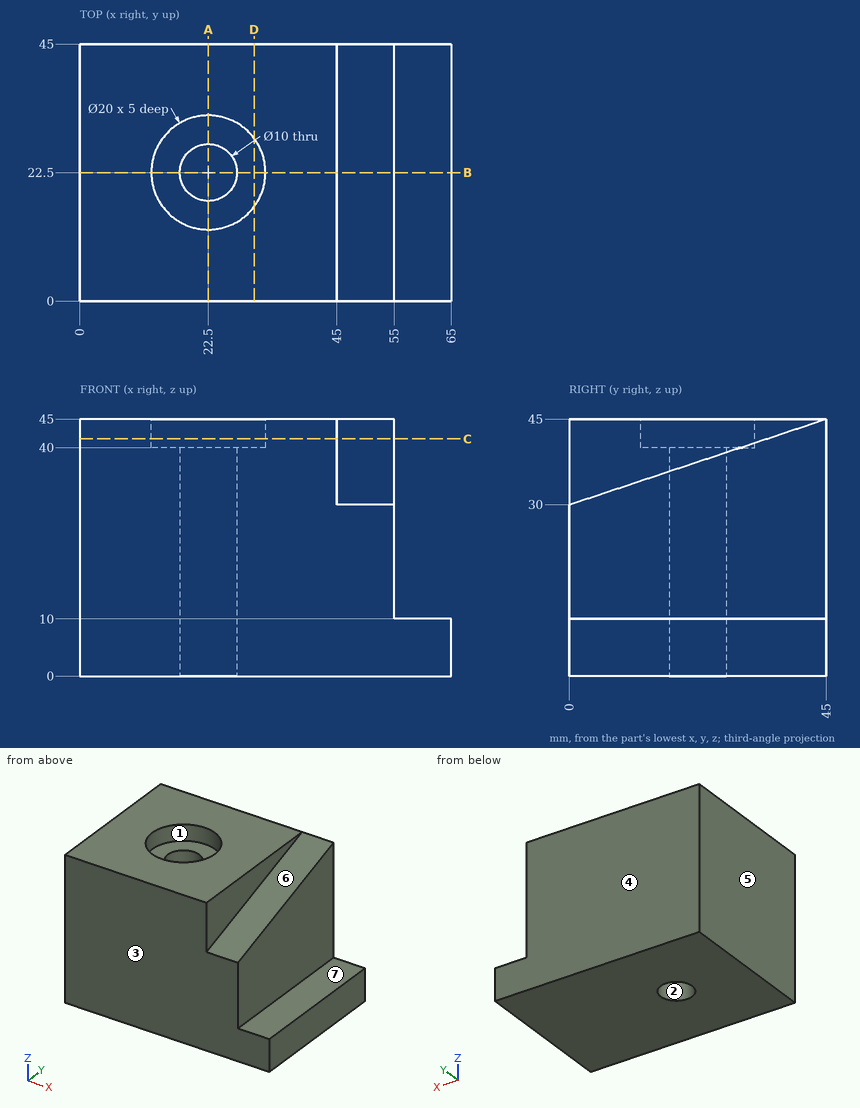
Could you check a few things on this drawing? It's one solid part, dimensions in mm from its lowest x, y, z. A direction names the side the tool comes from. Round coordinates to 2 decimals unless told otherwise and drop trailing zeros. Order: outer loops, then holes, each group sorted by start corner. A loop starts at its lowest first (then second) coordinate and runs counter-clockwise, first axis right, second up. Notation, with made-up numbers: M 87,-37 L 144,-37 A13 ccw 144,-19 Z; hole C -14.75,-33.5 d4. An arc over 180 degrees is marked long. Use a Markdown table: item, result.
1) Imagine slicing it at D-D (x = 30.5). List the corners of the cut face in (y, z) for me, then the cut area to 4 significant figures.
Geometry says:
| item | result |
|---|---|
| outline | M 0,0 L 45,0 L 45,45 L 28.5,45 L 28.5,40 L 16.5,40 L 16.5,45 L 0,45 Z |
| area | 1,965 mm² |
2) Imagine slicing it at A-A (x = 22.5). List the corners of the cut face in (y, z) for me.
Geometry says:
| item | result |
|---|---|
| outline | M 0,0 L 17.5,0 L 17.5,40 L 12.5,40 L 12.5,45 L 0,45 Z; M 27.5,0 L 45,0 L 45,45 L 32.5,45 L 32.5,40 L 27.5,40 Z |
3) On a 3-axis mill with a long thin cutter (end or side, diameter ignored), from which of +Z, -Z, +X, -X, +Y, -Y can I reach the whole of each face in a straight line? I mean the marked faces 5, 6 and 7. Say none if no direction works.
Geometry says:
| item | result |
|---|---|
| face 5 | +Z, -Z, -X, +Y, -Y |
| face 6 | +Z, +X, -Y |
| face 7 | +Z, +X, +Y, -Y |
4) Imagine slicing it at B-B (y = 22.5). List the corners of the cut face in (x, z) for me.
Geometry says:
| item | result |
|---|---|
| outline | M 0,0 L 17.5,0 L 17.5,40 L 12.5,40 L 12.5,45 L 0,45 Z; M 27.5,0 L 65,0 L 65,10 L 55,10 L 55,37.5 L 45,37.5 L 45,45 L 32.5,45 L 32.5,40 L 27.5,40 Z |
5) I'm going to push flat-ended pins straight in: P1, Ø12, axis at y = 4.5, z = 29.5, coming from the -X side; P2, Ø16, axis at x = 22.5, y = 22.5, coming from the +Z side; P3, Ø10.5, axis at y = 33, z = 26, coming from the +X side; P4, Ø3, axis at x = 60, y = 29, coming from the +Z side. Where does each tip first touch, or does it pass through?
Geometry says:
| item | result |
|---|---|
| P1 | stops at x = 0 |
| P2 | stops at z = 40 |
| P3 | stops at x = 55 |
| P4 | stops at z = 10 |
6) If I drill on line 1 along Y through (x, z) = (22.5, 41.95); line 2 along Y through (x, z) = (22.5, 19.5); line 3 along X through (y, z) = (22, 43), over which ranges is the centre line in solid material (lowest first)?
Geometry says:
| item | result |
|---|---|
| line 1 | y = 0 to 12.5, 32.5 to 45 |
| line 2 | y = 0 to 17.5, 27.5 to 45 |
| line 3 | x = 0 to 12.51, 32.49 to 45 |
7) If we mould it in two halves opening along Y, with no side actions, what happens to the marked faces 1, 2, 3 and 4? For each: +Y half, -Y half, draft (parallel to the pull), parting line (faces both ways), or undercut.
Geometry says:
| item | result |
|---|---|
| face 1 | undercut |
| face 2 | undercut |
| face 3 | -Y half |
| face 4 | +Y half |
8) Imagine slicing it at C-C (z = 41.5). List the corners of the cut face in (x, y) for me.
Geometry says:
| item | result |
|---|---|
| outline | M 0,0 L 45,0 L 45,34.5 L 55,34.5 L 55,45 L 0,45 Z; hole C 22.5,22.5 d20 |
